Read the model definition and answer for the solid it produces. Units are mm, in the model's axes. A direction names the side the tool comes from. Coordinates: 2 decimals unless noted, no trailing zeros. Write each loop counter-clockwise with the first axis right and the second up, starting at its lowest first coordinate (ties: lowest second). Pieces come first, ordered by that corner, then holes. Notation, with made-up numbers: (37.5, -15) -> (75.5, -15) arc R16 cw to (75.5, 0) -> close; hole circle Ø10 at (7, -25.5). An arc over 180 degrees is marked (long way). Answer in a Markdown table with one row per item. Add a question column.
Item 1: Section A-A on x = 6.5 is taken. Write down the section's boundary in (y, z).
Item 2: Given pin 1 Ø0.6 at (y, z) = (0.5, -1) entering from -X; pin 2 Ø1 at (x, z) = (4.5, -0.5) entering from -Y; pin 3 Ø1.5 at (x, z) = (2.5, 1.5) entering from +Y; pin 4 Ø2 at (x, z) = (4.5, -1.5) entering from +Y, each flat-ended and moving along its own axis, determine where each tip first touches the part or whether it passes through.
Item 3: Which of the six approach directions +Z, -Z, +X, -X, +Y, -Y give full straight-line access (tool end or side, diameter ignored) to faces 1 (the face through (0.54, -0.86, 0.51)), 2 (the face through (0, 0, -1.2)), 3 (the face through (5.865, -0.195, 1.487))?
Item 4: Straight lines are drawn through the part: line 1 (Z direction, x = 7, y = 0.05); line 2 (Z direction, x = 1.5, y = -0.2); line 3 (Y direction, x = 1, z = -1.35). For each, find the intervals that lie inside material, in ascending order. Write a range as from..to.
Item 5: For a pull along Z with two mould halves and no side action, classify faces 4 (the face through (10, 0, 0)), 5 (the face through (0.54, 0.86, -0.51)), 6 (the face through (0.35, -0.58, -2.61)) as +Z half, -Z half, draft (parallel to the pull), parting line (faces both ways), or undercut.
```python
from build123d import *

# Parameters (mm, degrees)
FILLET1_R   = 0.1
HEX_2_DEPTH = 1.1


with BuildPart() as part:
    # BodySke → BaseBody (revolve)
    with BuildSketch(Plane.XY):
        Polygon((0, 0), (0, 2.675), (0.685, 2.675), (1.86, 1.5), (9.7195, 1.5), (10, 1.2195), (10, 0), align=None)
    revolve(axis=Axis((0, 0, 0), (1, 0, 0)))

    # Fillet1
    fillet1_edges = [part.edges().sort_by_distance(p)[0] for p in [
        (1.86, -1.5, 0),
    ]]
    fillet(fillet1_edges, radius=FILLET1_R)

    # Sketch2 → PreBroach (revolve, cut)
    with BuildSketch(Plane.XY):
        Polygon((0, 1), (1.1, 1), (1.677350269, 0), (0, 0), align=None)
    revolve(axis=Axis((0, 0, 0), (1, 0, 0)), mode=Mode.SUBTRACT)

    # Sketch3 → Hex 2 (cut)
    with BuildSketch(Plane.ZY):
        Polygon((-1, -0.577350269), (-1, 0.577350269), (0, 1.154700538), (1, 0.577350269), (1, -0.577350269), (0, -1.154700538), align=None)
    extrude(amount=-HEX_2_DEPTH, mode=Mode.SUBTRACT)


solid = part.part
```
Results below:
| question | item | result |
|---|---|---|
| 1 | outline | circle Ø3 at (0, 0) |
| 2 | pin 1 | stops at x = 0 |
| 2 | pin 2 | stops at y = -1.5 |
| 2 | pin 3 | stops at y = 1.3 |
| 2 | pin 4 | stops at y = 1.41 |
| 3 | face 1 | -X |
| 3 | face 2 | +Z, -Z, -X, +Y, -Y |
| 3 | face 3 | +X |
| 4 | line 1 | z = -1.5..1.5 |
| 4 | line 2 | z = -1.85..-0.23, 0.23..1.85 |
| 4 | line 3 | y = -1.94..1.94 |
| 5 | face 4 | draft |
| 5 | face 5 | undercut |
| 5 | face 6 | parting line |
